Here's how the part is built. I have some questions about the finished solid (model axes, mm). Face numbers are marked on the shaded views. A direction names the side the tool comes from. Round coordinates to 2 decimals unless told otherwise and drop trailing zeros. Order: outer loops, then holes, each group sorted by start corner. A loop starts at its lowest first (then second) coordinate and runs counter-clockwise, first axis right, second up. Notation, with made-up numbers: (62, 50.5) - (119, 50.5) arc R27 ccw to (119, 89.5) - close; hole circle Ø1 at (-8.5, 80.5). An arc over 180 degrees is marked (long way). One line per item, written item: value.
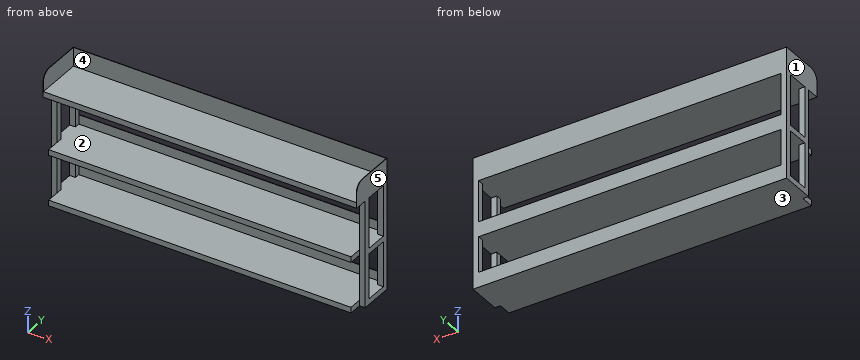
from build123d import *

# Parameters (mm, degrees)
F0_W           = 1670
F0_H           = 250
F1_DEPTH       = 30
F2_W           = 30
F2_H           = 30
F3_DEPTH       = 570
F4_W           = 250
F4_H           = 30
F5_DEPTH       = 805
F5_DEPTH_BACK  = 805
F7_DEPTH       = 100
F8_R           = 50
F9_W           = 1610
F9_H           = 2
F10_DEPTH      = 50
F11_W          = 1610
F11_H          = 2
F12_DEPTH      = 50
F13_W          = 30
F13_H          = 30
F14_DEPTH      = 25
F14_DEPTH_BACK = 95


with BuildPart() as f1:
    # F0 (on Top) → F1 (new body)
    with BuildSketch(Plane.XY):
        Rectangle(F0_W, F0_H)
    extrude(amount=F1_DEPTH)

    # F2 (on face) → F3 (join)
    with BuildSketch(Plane(origin=(0, 0, 0), x_dir=(1, 0, 0), z_dir=(0, 0, -1))):
        with Locations((-820, 40)):
            Rectangle(F2_W, F2_H)
        with Locations((820, 40)):
            Rectangle(F2_W, F2_H)
        with Locations((820, -110)):
            Rectangle(F2_W, F2_H)
        with Locations((-820, -110)):
            Rectangle(F2_W, F2_H)
    extrude(amount=F3_DEPTH)

    # F4 (on Right) → F5 (join, two sides)
    with BuildSketch(Plane.YZ) as f5_sk:
        with Locations((0, -285)):
            Rectangle(F4_W, F4_H)
        with Locations((0, -555)):
            Rectangle(F4_W, F4_H)
    extrude(amount=F5_DEPTH)
    extrude(f5_sk.sketch, amount=-F5_DEPTH_BACK)

    # F6 (on face) → F7 (join)
    with BuildSketch(Plane.XY.offset(30)):
        Polygon((-835, 125), (-835, -125), (-833, -125), (-833, 123), (833, 123), (833, -125), (835, -125), (835, 125), align=None)
    extrude(amount=F7_DEPTH)

    # F8
    f8_edges = [f1.edges().sort_by_distance(p)[0] for p in [
        (-834, -125, 130),
        (834, -125, 130),
    ]]
    fillet(f8_edges, radius=F8_R)

    # F9 (on face) → F10 (join)
    with BuildSketch(Plane.XY.offset(-270)):
        with Locations((0, 124)):
            Rectangle(F9_W, F9_H)
    extrude(amount=F10_DEPTH)

    # F11 (on face) → F12 (join)
    with BuildSketch(Plane.XY.offset(-540)):
        with Locations((0, 124)):
            Rectangle(F11_W, F11_H)
    extrude(amount=F12_DEPTH)

    # F13 (on Front) → F14 (join, two sides)
    with BuildSketch(Plane.XZ) as f14_sk:
        with Locations((820, -285)):
            Rectangle(F13_W, F13_H)
        with Locations((820, -555)):
            Rectangle(F13_W, F13_H)
        with Locations((-820, -555)):
            Rectangle(F13_W, F13_H)
        with Locations((-820, -285)):
            Rectangle(F13_W, F13_H)
    extrude(amount=F14_DEPTH)
    extrude(f14_sk.sketch, amount=-F14_DEPTH_BACK)


solid = f1.part
Q1. Will these pins go through, and if not, where does the flat tip stop? pin 1 (24 mm diameter, centred on y = -86.5, z = -560, fed in from +X); pin 2 (9 mm diameter, centred on y = -94, z = -290.5, fed in from -X); pin 3 (9 mm diameter, centred on x = 824.5, z = -198.5, fed in from -Y).
Results list:
pin 1: x = 805
pin 2: x = -805
pin 3: y = -55
Q2. If I drill on line 1 along Z through (x, y) = (-500, 10.5); line 2 along X through (y, z) = (106.5, -353); line 3 along X through (y, z) = (111, 75), over which ranges is the centre line in solid material (lowest first)?
Results list:
line 1: -570 to -540, -300 to -270, 0 to 30
line 2: -835 to -805, 805 to 835
line 3: -835 to -833, 833 to 835
Q3. If we section it at B-B, the plane x = -379.5: Please give me the cut outline in (y, z), then the cut area to 3 significant figures.
Results list:
outline: (-125, -570) - (125, -570) - (125, -490) - (123, -490) - (123, -540) - (-125, -540) - close; (-125, -300) - (125, -300) - (125, -220) - (123, -220) - (123, -270) - (-125, -270) - close; (-125, 0) - (125, 0) - (125, 130) - (123, 130) - (123, 30) - (-125, 30) - close
area: 22,900 mm²
Q4. We'd pull the mould along X, two halves only. Please class the marked faces 1, 2 and 3: released by +X, released by -X, zero draft, split by the parting line, or undercut.
Results list:
face 1: released by -X
face 2: undercut
face 3: zero draft
Q5. If we section it at D-D, the plane z = -104: Please give me the cut outline in (x, y).
Results list:
outline: (-835, -55) - (-805, -55) - (-805, -25) - (-835, -25) - close; (-835, 95) - (-805, 95) - (-805, 125) - (-835, 125) - close; (805, -55) - (835, -55) - (835, -25) - (805, -25) - close; (805, 95) - (835, 95) - (835, 125) - (805, 125) - close
Q6. If we section it at C-C, the plane y = 14: Please give me the cut outline in (x, z).
Results list:
outline: (-835, -570) - (835, -570) - (835, -540) - (-835, -540) - close; (-835, -300) - (835, -300) - (835, -270) - (-835, -270) - close; (-835, 0) - (835, 0) - (835, 130) - (833, 130) - (833, 30) - (-833, 30) - (-833, 130) - (-835, 130) - close
Q7. If we section it at A-A, the plane z = -236.5: Please give me the cut outline in (x, y).
Results list:
outline: (-835, -55) - (-805, -55) - (-805, -25) - (-835, -25) - close; (-835, 95) - (-805, 95) - (-805, 123) - (805, 123) - (805, 95) - (835, 95) - (835, 125) - (-835, 125) - close; (805, -55) - (835, -55) - (835, -25) - (805, -25) - close
Q8. Which directions (+Z, -Z, +X, -X, +Y, -Y) give clear straight access to the entire face, cutting with the end or side of a thin tool? Please do the marked faces 4 and 5.
Results list:
face 4: +Z, -Y
face 5: +Z, -Z, +X, +Y, -Y
